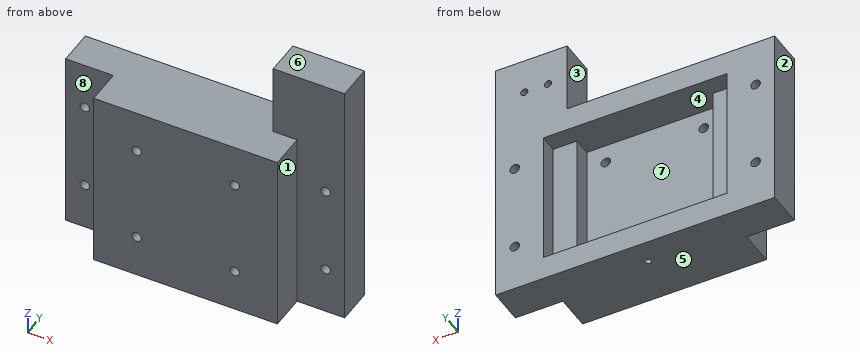
from build123d import *

# Parameters (mm, degrees)
CROQUIS1_W              = 77.15
CROQUIS1_H              = 77.15
SALIENTE_EXTRUIR1_DEPTH = 15
CROQUIS4_W              = 10
CROQUIS4_H              = 77.15
SALIENTE_EXTRUIR2_DEPTH = 7.5
CROQUIS4_3_W            = 20
CROQUIS4_3_H            = 77.15
SALIENTE_EXTRUIR3_DEPTH = 15
SALIENTE_EXTRUIR4_DEPTH = 10
CROQUIS7_R              = 2
CORTAR_EXTRUIR2_DEPTH   = 50
CROQUIS8_R              = 2
CORTAR_EXTRUIR3_DEPTH   = 40
CROQUIS9_W              = 117.15
CROQUIS9_H              = 15
SALIENTE_EXTRUIR5_DEPTH = 30
CROQUIS10_W             = 87.15
CROQUIS10_H             = 30
CORTAR_EXTRUIR4_DEPTH   = 40
CROQUIS11_R             = 1.5
CORTAR_EXTRUIR5_DEPTH   = 10
CROQUIS12_R             = 1.25
CORTAR_EXTRUIR6_DEPTH   = 4.3


with BuildPart() as part:
    # Croquis1 → Saliente-Extruir1 (new body)
    with BuildSketch(Plane(origin=(0, 0, 0), x_dir=(1, 0, 0), z_dir=(0, 1, 0))):
        Rectangle(CROQUIS1_W, CROQUIS1_H)
    extrude(amount=SALIENTE_EXTRUIR1_DEPTH)

    # Croquis4 → Saliente-Extruir2 (add)
    with BuildSketch(Plane(origin=(0, 15, 0), x_dir=(1, 0, 0), z_dir=(0, 1, 0))):
        with Locations((-33.575, 0)):
            Rectangle(CROQUIS4_W, CROQUIS4_H)
    saliente_extruir2 = extrude(amount=SALIENTE_EXTRUIR2_DEPTH)

    # Croquis4_3 → Saliente-Extruir3 (add)
    with BuildSketch(Plane(origin=(0, 15, 0), x_dir=(1, 0, 0), z_dir=(0, 1, 0))):
        with Locations((-48.575, 0)):
            Rectangle(CROQUIS4_3_W, CROQUIS4_3_H)
    saliente_extruir3 = extrude(amount=SALIENTE_EXTRUIR3_DEPTH)

    # Simetr_a1: Saliente-Extruir2, Saliente-Extruir3 across plane
    add(saliente_extruir2.mirror(Plane.ZY))
    add(saliente_extruir3.mirror(Plane.ZY))

    # Croquis5 → Saliente-Extruir4 (add)
    with BuildSketch(Plane.XY.offset(38.575)):
        Polygon((-58.575, 30), (-38.575, 30), (38.575, 30), (58.575, 30), (58.575, 15), (38.575, 15), (38.575, 0), (-38.575, 0), (-38.575, 15), (-58.575, 15), align=None)
    saliente_extruir4 = extrude(amount=-SALIENTE_EXTRUIR4_DEPTH)

    # Croquis7 → Cortar-Extruir2 (cut)
    with BuildSketch(Plane(origin=(0, 15, 0), x_dir=(1, 0, 0), z_dir=(0, 1, 0))):
        with Locations(Location((20.575, 20.575, 0), (0, 0, 270))):
            Circle(CROQUIS7_R)
        with Locations(Location((-20.575, 20.575, 0), (0, 0, 270))):
            Circle(CROQUIS7_R)
        with Locations(Location((20.575, -20.575, 0), (0, 0, 270))):
            Circle(CROQUIS7_R)
        with Locations(Location((-20.575, -20.575, 0), (0, 0, 270))):
            Circle(CROQUIS7_R)
    extrude(amount=-CORTAR_EXTRUIR2_DEPTH, mode=Mode.SUBTRACT)

    # Croquis8 → Cortar-Extruir3 (cut)
    with BuildSketch(Plane(origin=(0, 30, 0), x_dir=(1, 0, 0), z_dir=(0, 1, 0))):
        with Locations(Location((50.575, 18.575, 0), (0, 0, 270))):
            Circle(CROQUIS8_R)
        with Locations(Location((50.575, -18.575, 0), (0, 0, 270))):
            Circle(CROQUIS8_R)
        with Locations(Location((-50.575, 18.575, 0), (0, 0, 270))):
            Circle(CROQUIS8_R)
        with Locations(Location((-50.575, -18.575, 0), (0, 0, 270))):
            Circle(CROQUIS8_R)
    extrude(amount=-CORTAR_EXTRUIR3_DEPTH, mode=Mode.SUBTRACT)

    # Simetr_a2: Saliente-Extruir4 across plane
    add(saliente_extruir4.mirror(Plane(origin=(0, 0, 0), x_dir=(1, 0, 0), z_dir=(0, 0, -1))))

    # Croquis9 → Saliente-Extruir5 (add)
    with BuildSketch(Plane.XY.offset(38.575)):
        with Locations((0, 22.5)):
            Rectangle(CROQUIS9_W, CROQUIS9_H)
    extrude(amount=SALIENTE_EXTRUIR5_DEPTH)

    # Croquis10 → Cortar-Extruir4 (cut)
    with BuildSketch(Plane(origin=(0, 30, 0), x_dir=(1, 0, 0), z_dir=(0, 1, 0))):
        with Locations((-15, -53.575)):
            Rectangle(CROQUIS10_W, CROQUIS10_H)
    extrude(amount=-CORTAR_EXTRUIR4_DEPTH, mode=Mode.SUBTRACT)

    # Croquis11 → Cortar-Extruir5 (cut)
    with BuildSketch(Plane(origin=(0, 30, 0), x_dir=(1, 0, 0), z_dir=(0, 1, 0))):
        with Locations(Location((36.575, -53.575, 0), (0, 0, 270))):
            Circle(CROQUIS11_R)
        with Locations(Location((46.575, -53.575, 0), (0, 0, 270))):
            Circle(CROQUIS11_R)
    extrude(amount=-CORTAR_EXTRUIR5_DEPTH, mode=Mode.SUBTRACT)

    # Croquis12 → Cortar-Extruir6 (cut)
    with BuildSketch(Plane(origin=(0, 0, -38.575), x_dir=(-1, 0, 0), z_dir=(0, 0, -1))):
        with Locations((0, 20)):
            Circle(CROQUIS12_R)
    extrude(amount=-CORTAR_EXTRUIR6_DEPTH, mode=Mode.SUBTRACT)


solid = part.part
Read the model definition and answer for the solid it produces. Units are mm, in the model's axes. Face numbers are marked on the shaded views. A direction names the side the tool comes from. Give positions to 0.01 mm unless a question says otherwise; leave off trailing zeros. Write each loop counter-clockwise with the first axis right and the second up, starting at its lowest first coordinate (ties: lowest second). Pieces come first, ordered by that corner, then holes. Notation, with made-up numbers: (44, 13.25) - (94, 13.25) arc R21 cw to (94, 46.25) - close; hole circle Ø1 at (25, -28). An arc over 180 degrees is marked (long way). Return JSON: item names as keys, results as strings.
Q1. For a pull along Z with two mould halves and no side action, classify the marked faces 5, 6, 7 and 8 as released by +Z, released by -Z, zero draft, split by the parting line, or undercut.
Reply:
{"face 5": "released by -Z", "face 6": "released by +Z", "face 7": "undercut", "face 8": "zero draft"}
Q2. A cutting plane is placed at D-D, the plane z = 32. Determine the outline of the cut face in (x, y) (3 decimals), and give its area (3 significant figures).
Reply:
{"outline": "(-58.575, 15) - (-38.575, 15) - (-38.575, 0) - (38.575, 0) - (38.575, 15) - (58.575, 15) - (58.575, 30) - (-58.575, 30) - close", "area": "2,910 mm²"}
Q3. A cutting plane is placed at C-C, the plane x = -4. Determine the outline of the cut face in (y, z) (3 decimals).
Reply:
{"outline": "(0, -38.575) - (30, -38.575) - (30, -28.575) - (15, -28.575) - (15, 28.575) - (30, 28.575) - (30, 38.575) - (0, 38.575) - close"}
Q4. Consider line 1 along X through (y, z) = (11, -20.5) (3 decimals); line 2 along X through (y, z) = (19, -17) (3 decimals); line 3 along Z through (x, y) = (22, 23.25) (3 decimals). Determine where each line is inside the solid, lowest interval first. Write a range as [from, to].
Reply:
{"line 1": "[-38.575, -22.574], [-18.576, 18.576], [22.574, 38.575]", "line 2": "[-58.575, -51.808], [-49.342, -28.575], [28.575, 49.342], [51.808, 58.575]", "line 3": "[-38.575, -28.575], [28.575, 38.575]"}
Q5. For the marked faces 1, 2, 3 and 4, determine the directions among +Z, -Z, +X, -X, +Y, -Y from which every point of the face is accessible in a straight line to the end or side of a thin tool.
Reply:
{"face 1": "+Z, -Z, +X, -Y", "face 2": "+Z, -Z, -X, +Y, -Y", "face 3": "+Z, -X, +Y, -Y", "face 4": "+Y"}
Q6. Given P1, Ø0.9, axis at x = 47, z = 53, coming from the +Y side; P2, Ø1, axis at y = 10.5, z = -6, coming from the +X side (3 decimals); P3, Ø2, axis at x = 0, y = 20, coming from the -Z side (3 decimals); P4, Ø3, axis at x = -20.575, z = 20.575, coming from the -Y side, each flat-ended and moving along its own axis, determine where each tip first touches the part or whether it passes through.
Reply:
{"P1": "y = 20", "P2": "x = 38.575", "P3": "z = -34.275", "P4": "through"}
Q7. A cutting plane is placed at B-B, the plane z = -2. Determine the outline of the cut face in (x, y) (3 decimals), and give its area (3 significant figures).
Reply:
{"outline": "(-58.575, 15) - (-38.575, 15) - (-38.575, 0) - (38.575, 0) - (38.575, 15) - (58.575, 15) - (58.575, 30) - (38.575, 30) - (38.575, 22.5) - (28.575, 22.5) - (28.575, 15) - (-28.575, 15) - (-28.575, 22.5) - (-38.575, 22.5) - (-38.575, 30) - (-58.575, 30) - close", "area": "1,910 mm²"}
Q8. A cutting plane is placed at A-A, the plane y = 8.75. Determine the outline of the cut face in (x, z) (3 decimals).
Reply:
{"outline": "(-38.575, -38.575) - (38.575, -38.575) - (38.575, 38.575) - (-38.575, 38.575) - close; hole circle Ø4 at (-20.575, -20.575); hole circle Ø4 at (-20.575, 20.575); hole circle Ø4 at (20.575, -20.575); hole circle Ø4 at (20.575, 20.575)"}
